from build123d import *

# Parameters (mm, degrees)
EXTRUDE_1_DEPTH        = 14
EXTRUDE_2_DEPTH        = 7
CUT_EXTRUDE_1_DEPTH    = 41.028932
CUT_EXTRUDE_2_DEPTH    = 38.1
HOLE_WIZARD_M4_1_D     = 4.318
HOLE_WIZARD_M4_1_DEPTH = 14
FILLET_1_R             = 5
FILLET_3_R             = 1.27
FILLET_4_R             = 1.27


with BuildPart() as part:
    # 草图1 → 凸台-拉伸1 (new body)
    with BuildSketch(Plane.XZ.offset(15)):
        Polygon((4.743453, -52.27499), (35.219756, -21.798688), (-2.928932, 16.35), (-41.028932, 16.35), (-41.028932, -16.35), align=None)
    extrude(amount=-EXTRUDE_1_DEPTH)

    # 草图2 → 凸台-拉伸2 (add)
    with BuildSketch(Plane.XZ.offset(15)):
        Polygon((43.705037, -23.212901), (38.75529, -18.263154), (35.219756, -21.798688), (28.148688, -28.869756), (33.098435, -33.819503), align=None)
    extrude(amount=-EXTRUDE_2_DEPTH)

    # 草图3 → 切除-拉伸1 (cut)
    with BuildSketch(Plane.ZY.offset(41.028932)):
        with BuildLine():
            Line((5.5795, -1), (-6.270766, -1))
            ThreePointArc((-6.270766, -1), (-0.345633, -6.055118), (5.5795, -1))
        make_face()
    extrude(amount=-CUT_EXTRUDE_1_DEPTH, mode=Mode.SUBTRACT)

    # 草图4 → 切除-拉伸2 (cut)
    with BuildSketch(Plane(origin=(6.710534, 0, 6.710534), x_dir=(0.707107, 0, -0.707107), z_dir=(0.707107, 0, 0.707107))):
        with BuildLine():
            Line((29.445831, -1), (9.538252, -1))
            ThreePointArc((9.538252, -1), (19.492041, -10.039754), (29.445831, -1))
        make_face()
    extrude(amount=-CUT_EXTRUDE_2_DEPTH, mode=Mode.SUBTRACT)

    # M4 间隙孔1
    with Locations(Plane(origin=(0, -15, 0), x_dir=(-1, 0, 0), z_dir=(0, -1, 0))):
        with Locations((35.028932, -10.35), (-5, 0), (15, 15), (12.103043, -10.35), (35.028932, 10.35), (-4.743453, 43.789709), (-26.734474, 21.798688)):
            Hole(HOLE_WIZARD_M4_1_D / 2, depth=HOLE_WIZARD_M4_1_DEPTH)

    # 圆角1
    fillet_1_edges = [part.edges().sort_by_distance(p)[0] for p in [
        (-41.028932, -8, -16.35),
        (-41.028932, -8, 16.35),
        (-2.928932, -8, 16.35),
        (4.743453, -8, -52.27499),
    ]]
    fillet(fillet_1_edges, radius=FILLET_1_R)

    # 圆角3
    fillet_3_edges = [part.edges().sort_by_distance(p)[0] for p in [
        (31.684222, -8, -25.334222),
    ]]
    fillet(fillet_3_edges, radius=FILLET_3_R)

    # 圆角4
    fillet_4_edges = [part.edges().sort_by_distance(p)[0] for p in [
        (28.148688, -11.5, -28.869756),
    ]]
    fillet(fillet_4_edges, radius=FILLET_4_R)


solid = part.part
Model file for the job. Use its own axes, mm. A direction names the side the tool comes from. Give positions to 0.01 mm unless a question says otherwise; leave off trailing zeros. Loops run counter-clockwise (first coordinate to the right, second up) from the corner with the lowest first, then second, coordinate; pieces in that order, holes last.
1) Wall check: line 1 (X direction, y = -6.25, z = 12); line 2 (X direction, y = -5.5, z = 11); line 3 (Z direction, x = 1, y = -3.75). Give the ranges that are in metal, low to high.
2) Saw through at B-B (y = -4). Write the cut outline in (x, z).
3) Tool access for faces 5 (the flat face through (31.044, -11.549, -31.765)), 6 (the cylindrical face through (-20.802, -6.054, -0.464)), 7 (the cylindrical face through (-39.53, -7.9, 14.92)): list every direction of +Z, -Z, +X, -X, +Y, -Y with a clear straight run to the whole face (end or side of a thin tool).
4) Saw through at A-A (z = 10.35). Write the cut outline in (x, y), plus the area to 3 significant figures.
5) Saw through at D-D (x = 5.5). Count the separate pieces of the cut face and the enclosed holes in it, plus the area to 3 significant figures.
6) Pull direction X, two halves, no side cores. Call faces 1 (the flat face through (-9, -15, -17)), 2 (the cylindrical face through (31.436, -7.618, -26.095)), 3 (the cylindrical face through (6.994, -7.902, 0.827)), 4 (the flat face through (-41.029, -8, -1)): +X half, -X half, draft (parallel to the pull), parting line (faces both ways), or undercut.
7) Flat gauge pins, fed straight in: pin 1 Ø1.5 at (y, z) = (-3.5, 1.5) entering from -X; pin 2 Ø5 at (x, y) = (-5.5, -6) entering from -Z; pin 3 Ø1.5 at (x, y) = (-4, -7.5) entering from +Z. Where does each tip first touch, or does it go through?
8) Saw through at C-C (x = -28). Write the cut outline in (y, z), plus the area to 3 significant figures.
Answer block:
1. line 1: x = -40.99 to -36.42, -33.64 to -13.5, -10.71 to 1.42
1. line 2: x = -41.03 to -37.09, -32.97 to -14.16, -10.04 to 2.42
1. line 3: z = -49.34 to -39.7, -13.43 to 12.42
2. outline: (-41.03, -13.92) arc R5 ccw to (-39.12, -17.85) - (1.26, -49.54) arc R5 ccw to (7.88, -49.14) - (35.22, -21.8) - (26.99, -13.57) - (0.05, -40.51) - (-12.94, -27.52) - (14, -0.58) - (-1.46, 14.89) arc R5 ccw to (-5, 16.35) - (-36.03, 16.35) arc R5 ccw to (-41.03, 11.35) - (-41.03, 4.18) - (0, 4.18) - (0, -4.87) - (-41.03, -4.87) - close; hole circle Ø4.32 at (-35.03, -10.35); hole circle Ø4.32 at (-35.03, 10.35); hole circle Ø4.32 at (-15, -15); hole circle Ø4.32 at (-12.1, 10.35); hole circle Ø4.32 at (4.74, -43.79); hole circle Ø4.32 at (5, 0); hole circle Ø4.32 at (26.73, -21.8)
3. face 5: -Z, +Y, -Y
3. face 6: -X, +Y
3. face 7: +Z, -X, +Y, -Y
4. outline: (-41.03, -15) - (-37.19, -15) - (-37.19, -1) - (-41.03, -1) - close; (-32.87, -15) - (-14.26, -15) - (-14.26, -1) - (-32.87, -1) - close; (-9.94, -15) - (3.07, -15) - (3.07, -1) - (-9.94, -1) - close
4. area: 496 mm2
5. separate pieces: 3
5. enclosed holes: 0
5. area: 507 mm2
6. face 1: draft
6. face 2: +X half
6. face 3: undercut
6. face 4: -X half
7. pin 1: stops at x = 0
7. pin 2: stops at z = -46.2
7. pin 3: stops at z = 16.34
8. outline: (-15, -26.58) - (-1, -26.58) - (-1, -6.27) arc R6 cw to (-1, 5.58) - (-1, 16.35) - (-15, 16.35) - close
8. area: 556 mm2
